```python
from build123d import *

# Parameters (mm, degrees)
SKETCH1_W           = 162
SKETCH1_H           = 110
BOSS_EXTRUDE1_DEPTH = 55
SHELL1_T            = -5
BOSS_EXTRUDE3_DEPTH = 15
SKETCH6_W           = 17
SKETCH6_H           = 10.3
BOSS_EXTRUDE4_DEPTH = 3
SKETCH8_W           = 10
SKETCH8_H           = 5
BOSS_EXTRUDE5_DEPTH = 17.5
SKETCH9_W           = 25.3
SKETCH9_H           = 6.2
CUT_EXTRUDE1_DEPTH  = 5
SKETCH10_R          = 1.6
CUT_EXTRUDE2_DEPTH  = 11


with BuildPart() as part:
    # Sketch1 → Boss-Extrude1 (new, symmetric)
    with BuildSketch(Plane.XY):
        Rectangle(SKETCH1_W, SKETCH1_H)
    extrude(amount=BOSS_EXTRUDE1_DEPTH, both=True)

    # Shell1
    shell1_openings = [part.faces().sort_by_distance(p)[0] for p in [
        (0, 0, 55),
    ]]
    offset(amount=SHELL1_T, openings=shell1_openings, kind=Kind.INTERSECTION)

    # Sketch5 → Boss-Extrude3 (add, symmetric)
    with BuildSketch(Plane.XY):
        Polygon((-67.3, -55), (-67.3, -60.3), (-55.3, -60.3), (-55.3, -65.3), (-72.3, -65.3), (-72.3, -55), align=None)
        Polygon((67.3, -55), (67.3, -60.3), (55.3, -60.3), (55.3, -65.3), (72.3, -65.3), (72.3, -55), align=None)
    extrude(amount=BOSS_EXTRUDE3_DEPTH, both=True)

    # Sketch6 → Boss-Extrude4 (add)
    with BuildSketch(Plane(origin=(0, 0, -15), x_dir=(-1, 0, 0), z_dir=(0, 0, -1))):
        with Locations((63.8, -60.15)):
            Rectangle(SKETCH6_W, SKETCH6_H)
        with Locations((-63.8, -60.15)):
            Rectangle(SKETCH6_W, SKETCH6_H)
    extrude(amount=BOSS_EXTRUDE4_DEPTH)

    # Sketch8 → Boss-Extrude5 (add, symmetric)
    with BuildSketch(Plane(origin=(0, 0, 0), x_dir=(0, 0, -1), z_dir=(1, 0, 0))):
        with Locations((-60, 52.5)):
            Rectangle(SKETCH8_W, SKETCH8_H)
    extrude(amount=BOSS_EXTRUDE5_DEPTH, both=True)

    # Sketch9 → Cut-Extrude1 (cut)
    with BuildSketch(Plane(origin=(0, 55, 0), x_dir=(1, 0, 0), z_dir=(0, 1, 0))):
        with Locations((0, -59.1)):
            Rectangle(SKETCH9_W, SKETCH9_H)
    extrude(amount=-CUT_EXTRUDE1_DEPTH, mode=Mode.SUBTRACT)

    # Sketch10 → Cut-Extrude2 (cut)
    with BuildSketch(Plane.XY.offset(65)):
        with Locations((0, 52.5)):
            Circle(SKETCH10_R)
    extrude(amount=-CUT_EXTRUDE2_DEPTH, mode=Mode.SUBTRACT)


solid = part.part
```
Verification items for the finished model (mm, model axes). A direction names the side the tool comes from. Coordinates: 2 decimals unless noted, no trailing zeros. Write each loop counter-clockwise with the first axis right and the second up, starting at its lowest first coordinate (ties: lowest second). Pieces come first, ordered by that corner, then holes. Notation, with made-up numbers: (56, 54) - (61, 54) arc R20 cw to (61, 82) - close; hole circle Ø10 at (42, -39). An arc over 180 degrees is marked (long way). One line per question, with ' | ' between items. Start each with the question number.
1. Material ranges on line 1 along Y through (x, z) = (0, 54.75); line 2 along Y through (x, z) = (-66, 14.5); line 3 along X through (y, z) = (45.5, -12), recorded low to high.
2. Section check A-A (z = -12). Enter the section's corners in (x, y).
3. Draft check along Y on faces 6 (the flat face through (-61, -60.3, 0)), 7 (the flat face through (-55.3, -63, -1)), 8 (the flat face through (64, -65.3, -1)), 9 (the flat face through (-67.3, -58, 0)). Enter one of: released by +Y, released by -Y, zero draft, split by the parting line, or undercut.
4. Section check D-D (z = 43.5). Enter the section's corners in (x, y).
5. Access from +Z, -Z, +X, -X, +Y, -Y to the whole of each face (thin tool, end or side, straight path). Record for faces 1 (the flat face through (-17.5, 53, 60)), 2 (the flat face through (67.3, -58, 0)), 3 (the flat face through (-64, -60, -18)), 4 (the flat face through (-0.2, 54.8, 56)), 5 (the flat face through (17.5, 53, 60)).
6. Section check B-B (x = 42). Enter the section's corners in (y, z), plus the area to 3 significant figures.
7. Section check C-C (y = -23). Enter the section's corners in (x, z).
8. Gauge pin test, flat ends, axial feed: P1, Ø11.5, axis at x = 64.5, y = -60.5, coming from the +Z side; P2, Ø1.5, axis at y = 53, z = 57.5, coming from the -X side; P3, Ø5.5, axis at y = 53, z = 58, coming from the +X side; P4, Ø11.5, axis at x = -61.5, y = -59, coming from the -Z side. Record the tip position at first contact, or that the pin passes through.
Computed values:
1) line 1: -55 to -50, 50 to 50.9, 54.1 to 55 | line 2: -65.3 to -60.3, -55 to -50, 50 to 55 | line 3: -81 to -76, 76 to 81
2) outline: (-81, -55) - (-72.3, -55) - (-72.3, -65.3) - (-55.3, -65.3) - (-55.3, -60.3) - (-67.3, -60.3) - (-67.3, -55) - (67.3, -55) - (67.3, -60.3) - (55.3, -60.3) - (55.3, -65.3) - (72.3, -65.3) - (72.3, -55) - (81, -55) - (81, 55) - (-81, 55) - close; hole (-76, -50) - (76, -50) - (76, 50) - (-76, 50) - close
3) face 6: undercut | face 7: zero draft | face 8: released by -Y | face 9: undercut
4) outline: (-81, -55) - (81, -55) - (81, 55) - (-81, 55) - close; hole (-76, -50) - (76, -50) - (76, 50) - (-76, 50) - close
5) face 1: +Z, -X, +Y, -Y | face 2: +Z | face 3: -Z, +X, -X, -Y | face 4: +Y, -Y | face 5: +Z, +X, +Y, -Y
6) outline: (-55, -55) - (55, -55) - (55, 55) - (50, 55) - (50, -50) - (-50, -50) - (-50, 55) - (-55, 55) - close | area: 1,600 mm²
7) outline: (-81, -55) - (81, -55) - (81, 55) - (76, 55) - (76, -50) - (-76, -50) - (-76, 55) - (-81, 55) - close
8) P1: z = 55 | P2: x = -17.5 | P3: x = 17.5 | P4: z = -55
